```python
from build123d import *

# Parameters (mm, degrees)
BOSS_EXTRUDE1_DEPTH = 1
FILLET1_R           = 0.5


with BuildPart() as part:
    # Sketch1 → Boss-Extrude1 (new body)
    with BuildSketch(Plane.XY):
        with BuildLine():
            Line((0, 3.1), (5, 3.1))
            Line((5, 3.1), (5, 6.1))
            Line((5, 6.1), (-3.1, 6.1))
            ThreePointArc((-3.1, 6.1), (-9.2, 0), (-3.1, -6.1))
            Line((-3.1, -6.1), (5, -6.1))
            Line((5, -6.1), (5, -3.1))
            Line((5, -3.1), (0, -3.1))
            ThreePointArc((0, -3.1), (-3.1, 0), (0, 3.1))
        make_face()
    extrude(amount=BOSS_EXTRUDE1_DEPTH)

    # Fillet1
    fillet1_edges = [part.edges().sort_by_distance(p)[0] for p in [
        (0.95, 6.1, 0),
        (0.95, -6.1, 0),
        (0.95, 6.1, 1),
        (0.95, -6.1, 1),
        (-9.2, 0, 0),
        (-9.2, 0, 1),
    ]]
    fillet(fillet1_edges, radius=FILLET1_R - 0.0001)  # a hair under: the kernel refuses the full size


solid = part.part
```
For this review, take the finished solid that the model builds, in its own axes (mm). A direction names the side the tool comes from. Round coordinates to 2 decimals unless told otherwise and drop trailing zeros. Write each loop counter-clockwise with the first axis right and the second up, starting at its lowest first coordinate (ties: lowest second). Pieces come first, ordered by that corner, then holes. Notation, with made-up numbers: (28.5, 49.25) -> (81.5, 49.25) arc R20 ccw to (81.5, 88.25) -> close; hole circle Ø8 at (-31.5, 60). An arc over 180 degrees is marked (long way). One line per question, with ' | ' between items. Start each with the question number.
(1) Mouldability with a two-part tool opening along Y and no side actions: class faces 3 (the face through (5, 4.6, 0.5)), 4 (the face through (-3.1, -0.1, 0.5)) as released by +Y, released by -Y, zero draft, split by the parting line, or undercut.
(2) For line 1 along Y through (x, z) = (2, 0.65); line 2 along Y through (x, z) = (-1.5, 0.65); line 3 along X through (y, z) = (-1.5, 0.2), list the stretches that pass through material, from the lowest coordinate up. Write a range as from..to.
(3) Tool access review of faces 1 (the face through (2.5, 3.1, 0.5)), 2 (the face through (-3.5, 0.1, 1)): name each direction out of +Z, -Z, +X, -X, +Y, -Y from which nothing blocks a thin tool from reaching the whole face with its end or side.
(4) Add section C-C, the plane z = 0.8. Write out the cut boundary in (x, y), plus the area to 3 significant figures.
Answer list:
1) face 3: zero draft | face 4: undercut
2) line 1: -6.08..-3.1, 3.1..6.08 | line 2: -6.08..-2.71, 2.71..6.08 | line 3: -8.91..-2.71
3) face 1: +Z, -Z, +X | face 2: +Z, +X, -X, +Y, -Y
4) outline: (-3.1, -6) -> (5, -6) -> (5, -3.1) -> (0, -3.1) arc R3.1 cw to (0, 3.1) -> (5, 3.1) -> (5, 6) -> (-3.1, 6) arc R6 ccw to start | area: 108 mm²
